from build123d import *

# Parameters (mm, degrees)
F0_R     = 10.5
F0_R_2   = 9.125
F1_DEPTH = 40
F2_W     = 6
F2_H     = 35
F4_DEPTH = 3.5
F6_DEPTH = 25


with BuildPart() as f1:
    # F0 (on Top) → F1 (new body)
    with BuildSketch(Plane.XY):
        with BuildLine():
            Line((9.5, 10.6), (9.5, 12))
            Line((9.5, 12), (-9.5, 12))
            Line((-9.5, 12), (-9.5, 10.6))
            ThreePointArc((-9.5, 10.6), (-8.722183, 10.277817), (-8.4, 9.5))
            ThreePointArc((-8.4, 9.5), (-9.5, 8.4), (-10.6, 9.5))
            Line((-10.6, 9.5), (-12, 9.5))
            Line((-12, 9.5), (-12, -9.5))
            Line((-12, -9.5), (-10.6, -9.5))
            ThreePointArc((-10.6, -9.5), (-9.5, -8.4), (-8.4, -9.5))
            ThreePointArc((-8.4, -9.5), (-8.722183, -10.277817), (-9.5, -10.6))
            Line((-9.5, -10.6), (-9.5, -12))
            Line((-9.5, -12), (9.5, -12))
            Line((9.5, -12), (9.5, -10.6))
            ThreePointArc((9.5, -10.6), (8.722183, -8.722183), (10.6, -9.5))
            Line((10.6, -9.5), (12, -9.5))
            Line((12, -9.5), (12, 9.5))
            Line((12, 9.5), (10.6, 9.5))
            ThreePointArc((10.6, 9.5), (8.722183, 8.722183), (9.5, 10.6))
        make_face()
        Circle(F0_R, mode=Mode.SUBTRACT)
        Circle(F0_R)
        Circle(F0_R_2, mode=Mode.SUBTRACT)
        with BuildLine():
            Line((12, -12), (12, -9.5))
            Line((12, -9.5), (10.6, -9.5))
            ThreePointArc((10.6, -9.5), (10.277817, -10.277817), (9.5, -10.6))
            Line((9.5, -10.6), (9.5, -12))
            Line((9.5, -12), (12, -12))
        make_face()
        with BuildLine():
            Line((-10.6, -9.5), (-12, -9.5))
            Line((-12, -9.5), (-12, -12))
            Line((-12, -12), (-9.5, -12))
            Line((-9.5, -12), (-9.5, -10.6))
            ThreePointArc((-9.5, -10.6), (-10.277817, -10.277817), (-10.6, -9.5))
        make_face()
        with BuildLine():
            Line((-9.5, 10.6), (-9.5, 12))
            Line((-9.5, 12), (-12, 12))
            Line((-12, 12), (-12, 9.5))
            Line((-12, 9.5), (-10.6, 9.5))
            ThreePointArc((-10.6, 9.5), (-10.277817, 10.277817), (-9.5, 10.6))
        make_face()
        with BuildLine():
            Line((12, 9.5), (12, 12))
            Line((12, 12), (9.5, 12))
            Line((9.5, 12), (9.5, 10.6))
            ThreePointArc((9.5, 10.6), (10.277817, 10.277817), (10.6, 9.5))
            Line((10.6, 9.5), (12, 9.5))
        make_face()
        with BuildLine():
            Line((9.5, 9.5), (9.5, 10.6))
            ThreePointArc((9.5, 10.6), (8.722183, 8.722183), (10.6, 9.5))
            Line((10.6, 9.5), (9.5, 9.5))
        make_face()
        with BuildLine():
            ThreePointArc((10.6, 9.5), (10.277817, 10.277817), (9.5, 10.6))
            Line((9.5, 10.6), (9.5, 9.5))
            Line((9.5, 9.5), (10.6, 9.5))
        make_face()
        with BuildLine():
            Line((9.5, -9.5), (10.6, -9.5))
            ThreePointArc((10.6, -9.5), (8.722183, -8.722183), (9.5, -10.6))
            Line((9.5, -10.6), (9.5, -9.5))
        make_face()
        with BuildLine():
            ThreePointArc((9.5, -10.6), (10.277817, -10.277817), (10.6, -9.5))
            Line((10.6, -9.5), (9.5, -9.5))
            Line((9.5, -9.5), (9.5, -10.6))
        make_face()
        with BuildLine():
            Line((-9.5, -9.5), (-10.6, -9.5))
            ThreePointArc((-10.6, -9.5), (-10.277817, -10.277817), (-9.5, -10.6))
            Line((-9.5, -10.6), (-9.5, -9.5))
        make_face()
        with BuildLine():
            ThreePointArc((-8.4, -9.5), (-9.5, -8.4), (-10.6, -9.5))
            Line((-10.6, -9.5), (-9.5, -9.5))
            Line((-9.5, -9.5), (-9.5, -10.6))
            ThreePointArc((-9.5, -10.6), (-8.722183, -10.277817), (-8.4, -9.5))
        make_face()
        with BuildLine():
            ThreePointArc((-8.4, 9.5), (-8.722183, 10.277817), (-9.5, 10.6))
            Line((-9.5, 10.6), (-9.5, 9.5))
            Line((-9.5, 9.5), (-10.6, 9.5))
            ThreePointArc((-10.6, 9.5), (-9.5, 8.4), (-8.4, 9.5))
        make_face()
        with BuildLine():
            Line((-9.5, 9.5), (-9.5, 10.6))
            ThreePointArc((-9.5, 10.6), (-10.277817, 10.277817), (-10.6, 9.5))
            Line((-10.6, 9.5), (-9.5, 9.5))
        make_face()
    extrude(amount=F1_DEPTH)

    # F2 (on Front) → F3 (revolve, cut)
    with BuildSketch(Plane.XZ):
        with Locations((14, 20)):
            Rectangle(F2_W, F2_H)
    revolve(axis=Axis((0, 0, 16.744209), (0, 0, 1)), mode=Mode.SUBTRACT)

    # F0 (on Top) → F4 (join)
    with BuildSketch(Plane.XY):
        with BuildLine():
            Line((-9.5, 9.5), (-9.5, 10.6))
            ThreePointArc((-9.5, 10.6), (-10.277817, 10.277817), (-10.6, 9.5))
            Line((-10.6, 9.5), (-9.5, 9.5))
        make_face()
        with BuildLine():
            ThreePointArc((-8.4, 9.5), (-8.722183, 10.277817), (-9.5, 10.6))
            Line((-9.5, 10.6), (-9.5, 9.5))
            Line((-9.5, 9.5), (-10.6, 9.5))
            ThreePointArc((-10.6, 9.5), (-9.5, 8.4), (-8.4, 9.5))
        make_face()
        with BuildLine():
            Line((-9.5, -9.5), (-10.6, -9.5))
            ThreePointArc((-10.6, -9.5), (-10.277817, -10.277817), (-9.5, -10.6))
            Line((-9.5, -10.6), (-9.5, -9.5))
        make_face()
        with BuildLine():
            ThreePointArc((-8.4, -9.5), (-9.5, -8.4), (-10.6, -9.5))
            Line((-10.6, -9.5), (-9.5, -9.5))
            Line((-9.5, -9.5), (-9.5, -10.6))
            ThreePointArc((-9.5, -10.6), (-8.722183, -10.277817), (-8.4, -9.5))
        make_face()
        with BuildLine():
            Line((9.5, -9.5), (10.6, -9.5))
            ThreePointArc((10.6, -9.5), (8.722183, -8.722183), (9.5, -10.6))
            Line((9.5, -10.6), (9.5, -9.5))
        make_face()
        with BuildLine():
            ThreePointArc((9.5, -10.6), (10.277817, -10.277817), (10.6, -9.5))
            Line((10.6, -9.5), (9.5, -9.5))
            Line((9.5, -9.5), (9.5, -10.6))
        make_face()
        with BuildLine():
            Line((9.5, 9.5), (9.5, 10.6))
            ThreePointArc((9.5, 10.6), (8.722183, 8.722183), (10.6, 9.5))
            Line((10.6, 9.5), (9.5, 9.5))
        make_face()
        with BuildLine():
            ThreePointArc((10.6, 9.5), (10.277817, 10.277817), (9.5, 10.6))
            Line((9.5, 10.6), (9.5, 9.5))
            Line((9.5, 9.5), (10.6, 9.5))
        make_face()
    extrude(amount=-F4_DEPTH)

    # F5 (on face) → F6 (cut)
    with BuildSketch(Plane.XY.offset(40)):
        with BuildLine():
            Line((9.5, -9.5), (10.75, -9.5))
            ThreePointArc((10.75, -9.5), (8.616117, -8.616117), (9.5, -10.75))
            Line((9.5, -10.75), (9.5, -9.5))
        make_face()
        with BuildLine():
            ThreePointArc((9.5, -10.75), (10.383883, -10.383883), (10.75, -9.5))
            Line((10.75, -9.5), (9.5, -9.5))
            Line((9.5, -9.5), (9.5, -10.75))
        make_face()
        with BuildLine():
            Line((-9.5, 9.5), (-9.5, 10.75))
            ThreePointArc((-9.5, 10.75), (-10.383883, 10.383883), (-10.75, 9.5))
            Line((-10.75, 9.5), (-9.5, 9.5))
        make_face()
        with BuildLine():
            ThreePointArc((-8.25, -9.5), (-9.5, -8.25), (-10.75, -9.5))
            Line((-10.75, -9.5), (-9.5, -9.5))
            Line((-9.5, -9.5), (-9.5, -10.75))
            ThreePointArc((-9.5, -10.75), (-8.616117, -10.383883), (-8.25, -9.5))
        make_face()
        with BuildLine():
            Line((-9.5, -9.5), (-10.75, -9.5))
            ThreePointArc((-10.75, -9.5), (-10.383883, -10.383883), (-9.5, -10.75))
            Line((-9.5, -10.75), (-9.5, -9.5))
        make_face()
        with BuildLine():
            ThreePointArc((-8.25, 9.5), (-8.616117, 10.383883), (-9.5, 10.75))
            Line((-9.5, 10.75), (-9.5, 9.5))
            Line((-9.5, 9.5), (-10.75, 9.5))
            ThreePointArc((-10.75, 9.5), (-9.5, 8.25), (-8.25, 9.5))
        make_face()
        with BuildLine():
            Line((9.5, 9.5), (9.5, 10.75))
            ThreePointArc((9.5, 10.75), (8.616117, 8.616117), (10.75, 9.5))
            Line((10.75, 9.5), (9.5, 9.5))
        make_face()
        with BuildLine():
            ThreePointArc((10.75, 9.5), (10.383883, 10.383883), (9.5, 10.75))
            Line((9.5, 10.75), (9.5, 9.5))
            Line((9.5, 9.5), (10.75, 9.5))
        make_face()
    extrude(amount=-F6_DEPTH, mode=Mode.SUBTRACT)


solid = f1.part
Input: part model. Units: mm. Frame: model coordinates. A direction names the side the tool comes from. Round coordinates to 2 decimals unless told otherwise and drop trailing zeros. Write each loop counter-clockwise with the first axis right and the second up, starting at its lowest first coordinate (ties: lowest second). Pieces come first, ordered by that corner, then holes.
1) Cut plane B-B (x = -3.5). Return the cut outline in (y, z).
2) Contact query for flat-ended pins moving along their axis: P1, Ø1, axis at x = -1.5, z = 12, coming from the +Y side; P2, Ø3, axis at y = 5, z = 8, coming from the +X side; P3, Ø5, axis at x = 6, z = 7.5, coming from the -Y side; P4, Ø1.5, axis at x = 0.5, y = 8, coming from the +Z side. Output: stop coordinate, or through.
3) Draft query along Z for faces 1 (the flat face through (3, 11, 37.5)), 2 (the flat face through (0, -12, 39)), 3 (the flat face through (-10, 10, -3.5)). Return one class per face: pulls with the +Z half, pulls with the -Z half, needs draft (parallel to the pull), parting line crosses it, or undercut.
4) Ray query, L1, parallel to Y at x = 9.5, z = 39.3; L2, parallel to Y at x = 0, z = 14.5 (3 decimals). Return the intervals inside material, ascending.
5) Reachability of faces 4 (the cylindrical face through (-1.978, -8.908, 19.72)), 5 (the cylindrical face through (-2.38, -10.74, 20.24)), 6 (the flat face through (5, 8, 0)) from +Z, -Z, +X, -X, +Y, -Y: full face, straight path, thin tool, end or side. Return the list, or none.
6) Cut plane C-C (z = 13). Return the cut outline in (x, y) (3 decimals), then the cut area to 3 significant figures.
7) Cut plane A-A (y = 0). Return the cut outline in (x, z) (3 decimals).
Geometry says:
1. outline: (-12, 0) - (-8.43, 0) - (-8.43, 40) - (-12, 40) - (-12, 37.5) - (-10.43, 37.5) - (-10.43, 2.5) - (-12, 2.5) - close; (8.43, 0) - (12, 0) - (12, 2.5) - (10.43, 2.5) - (10.43, 37.5) - (12, 37.5) - (12, 40) - (8.43, 40) - close
2. P1: stops at y = 10.95
2. P2: stops at x = 10.43
2. P3: stops at y = -10.43
2. P4: passes through
3. face 1: undercut
3. face 2: needs draft
3. face 3: pulls with the -Z half
4. L1: y = -12 to -10.75, -8.25 to 8.25, 10.75 to 12
4. L2: y = -11 to -9.125, 9.125 to 11
5. face 4: +Z, -Z
5. face 5: none
5. face 6: -Z
6. outline: circle Ø22 at (0, 0); hole circle Ø18.25 at (0, 0)
6. area: 119 mm2
7. outline: (-12, 0) - (-9.125, 0) - (-9.125, 40) - (-12, 40) - (-12, 37.5) - (-11, 37.5) - (-11, 2.5) - (-12, 2.5) - close; (9.125, 0) - (12, 0) - (12, 2.5) - (11, 2.5) - (11, 37.5) - (12, 37.5) - (12, 40) - (9.125, 40) - close
